Part model, mm, in its own coordinate system. Round coordinates to 2 decimals unless told otherwise and drop trailing zeros. Write each loop counter-clockwise with the first axis right and the second up, starting at its lowest first coordinate (ties: lowest second). Pieces come first, ordered by that corner, then holes. Notation, with made-up numbers: M -2,-16 L 14,-16 A27 cw 14,5 Z; hole C -17,39.25 d8. An arc over 180 degrees is marked long. Use a Markdown table: item, result. Add a question column.
1) Drop flat-ended pins along their axis: P1, Ø15, axis at x = 14.5, z = 32, coming from the -Y side; P2, Ø3, axis at x = 13.5, y = 1, coming from the -Z side; P3, Ø12, axis at x = 31.5, y = 12.5, coming from the -Z side. Give the stop position or say it passes through.
2) Slice it at C-C on y = 0. Write the cut outline in (x, z).
3) Two-plate mould, pull along Y, no slides. Class faces 1 (the face through (25, 40, 26)), 2 (the face through (25, -60, 5)), 3 (the face through (50, 3, 21)), 4 (the face through (25, 50, 20)): released by +Y, released by -Y, zero draft, split by the parting line, or undercut.
4) Slice it at D-D on z = 26. Write the cut outline in (x, y), plus the area to 3 significant figures.
5) Wall check: probe 1 along Y at (x, z) = (4.5, 14); probe 2 along Y at (x, z) = (39, 15.5); probe 3 along Y at (x, z) = (32.5, 33.5). Give the ranges that are in metal, low to high.
6) Slice it at A-A on z = 7. Write the cut outline in (x, y) (3 decimals).
7) Slice it at B-B on x = 4.5. Write the cut outline in (y, z), plus the area to 3 significant figures.
```python
from build123d import *

# Parameters (mm, degrees)
F1_DEPTH = 50


# Not quite as in the source:
# - a feature names something its author has since deleted; it is built from what else it names


with BuildPart() as f1:
    # F0 (on Right) → F1 (new body)
    with BuildSketch(Plane.YZ):
        with BuildLine():
            Line((20.0000005408, 0), (50, 0))
            Line((50, 0), (50, 41))
            Line((50, 41), (40, 41))
            Line((40, 41), (40, 11))
            Line((40, 11), (27.9577328728, 10.8795773287))
            ThreePointArc((27.9577328728, 10.8795773287), (-0.2999844603, 29.9985001125), (-28.1697105934, 10.3183028941))
            Line((-28.1697105934, 10.3183028941), (-60, 10))
            Line((-60, 10), (-60, 0))
            Line((-60, 0), (-19.9999994592, 0))
            ThreePointArc((-19.9999994592, 0), (5.408e-07, 20), (20.0000005408, 0))
        make_face()
    extrude(amount=F1_DEPTH)


solid = f1.part
```
Entries:
| question | item | result |
|---|---|---|
| 1 | P1 | stops at y = -17.31 |
| 1 | P2 | stops at z = 19.84 |
| 1 | P3 | stops at z = 7.6 |
| 2 | outline | M 0,20 L 50,20 L 50,30 L 0,30 Z |
| 3 | face 1 | undercut |
| 3 | face 2 | released by -Y |
| 3 | face 3 | zero draft |
| 3 | face 4 | released by +Y |
| 4 | outline | M 0,-14.97 L 50,-14.97 L 50,14.97 L 0,14.97 Z; M 0,40 L 50,40 L 50,50 L 0,50 Z |
| 4 | area | 2,000 mm^2 |
| 5 | probe 1 | y = -26.53 to -14.28, 14.28 to 26.53, 40 to 50 |
| 5 | probe 2 | y = -25.69 to -12.64, 12.64 to 25.69, 40 to 50 |
| 5 | probe 3 | y = 40 to 50 |
| 6 | outline | M 0,-60 L 50,-60 L 50,-18.735 L 0,-18.735 Z; M 0,18.735 L 50,18.735 L 50,50 L 0,50 Z |
| 7 | outline | M -60,0 L -20,0 A20 cw 20,0 L 50,0 L 50,41 L 40,41 L 40,11 L 27.96,10.88 A30 ccw -28.17,10.32 L -60,10 Z |
| 7 | area | 1,620 mm^2 |
